Part model, mm, in its own coordinate system. A direction names the side the tool comes from. Round coordinates to 2 decimals unless told otherwise and drop trailing zeros. Order: outer loops, then holes, each group sorted by start corner. A loop starts at its lowest first (then second) coordinate and runs counter-clockwise, first axis right, second up. Notation, with made-up numbers: (-34.5, 61.5) -> (1.5, 61.5) arc R11 ccw to (1.5, 79.5) -> close; hole circle Ø3 at (44, 38.25). An arc over 180 degrees is marked (long way). Use CSV: the item, a comma, the result in double quotes.
```python
from build123d import *

# Parameters (mm, degrees)
EXTRUDE1_DEPTH     = 304.8
SKETCH2_R          = 1.5875
EXTRUDE2_DEPTH     = 1.5875
SKETCH3_R          = 1.5875
CUT_EXTRUDE3_DEPTH = 306.9883086
SKETCH6_R          = 1.5875
CUT_EXTRUDE5_DEPTH = 306.9883086
SKETCH7_W          = 17.4625
SKETCH7_H          = 11.77006403
CUT_EXTRUDE6_DEPTH = 306.893578563


with BuildPart() as part:
    # Sketch1 → Extrude1 (new body)
    with BuildSketch(Plane.XY):
        Polygon((0, 0), (0, 19.05), (-1.5875, 19.05), (-1.5875, 1.5875), (-19.05, 1.5875), (-19.05, 0), align=None)
    extrude(amount=EXTRUDE1_DEPTH)

    # Sketch2 → Extrude2 (cut)
    with BuildSketch(Plane(origin=(0, 0, 0), x_dir=(0, 0, -1), z_dir=(1, 0, 0))):
        with Locations((-298.45, 9.525)):
            Circle(SKETCH2_R)
        with Locations((-234.95, 9.525)):
            Circle(SKETCH2_R)
    extrude(amount=-EXTRUDE2_DEPTH, mode=Mode.SUBTRACT)

    # Sketch3 → Cut-Extrude3 (cut, through all)
    with BuildSketch(Plane(origin=(0, 0, 0), x_dir=(0, 0, -1), z_dir=(1, 0, 0))):
        with Locations((-26.555576272, 9.525)):
            Circle(SKETCH3_R)
        with Locations((-16.452788136, 9.525)):
            Circle(SKETCH3_R)
    extrude(amount=-CUT_EXTRUDE3_DEPTH, mode=Mode.SUBTRACT)

    # Sketch6 → Cut-Extrude5 (cut, through all)
    with BuildSketch(Plane(origin=(0, 0, 0), x_dir=(0, 0, -1), z_dir=(1, 0, 0))):
        with Locations((-8.59506403, 15.875)):
            Circle(SKETCH6_R)
        with Locations((-8.59506403, 3.175)):
            Circle(SKETCH6_R)
        with Locations((-6.35, 9.525)):
            Circle(SKETCH6_R)
    extrude(amount=-CUT_EXTRUDE5_DEPTH, mode=Mode.SUBTRACT)

    # Sketch7 → Cut-Extrude6 (cut, through all)
    with BuildSketch(Plane(origin=(0, 1.5875, 0), x_dir=(1, 0, 0), z_dir=(0, 1, 0))):
        with Locations((-10.31875, -5.885032015)):
            Rectangle(SKETCH7_W, SKETCH7_H)
    extrude(amount=-CUT_EXTRUDE6_DEPTH, mode=Mode.SUBTRACT)


solid = part.part
```
(1) Cut at A-A, the plane z = 157.5. Give the cut face in (x, y), then the cut area to 3 significant figures.
Reply:
outline,"(-19.05, 0) -> (0, 0) -> (0, 19.05) -> (-1.59, 19.05) -> (-1.59, 1.59) -> (-19.05, 1.59) -> close"
area,"58.0 mm2"
(2) Which spindle directions (+Z, -Z, +X, -X, +Y, -Y) get a long thin tool onto all of the face, cutting with end or side? Do faces 1 (the face through (-5, 1, 304.8)), 2 (the face through (-10, 1.588, 156)). Say none if no direction does.
Reply:
face 1,"+Z, +X, -X, +Y, -Y"
face 2,"+Z, -Z, -X, +Y"
(3) Probe probe 1 along Y at (x, z) = (-5, 194.5); probe 2 along X at (y, z) = (15, 234); probe 3 along Z at (x, y) = (-9.75, 1). List the from-to ranges inside material, lowest first. Write a range as [from, to].
Reply:
probe 1,"[0, 1.59]"
probe 2,"[-1.59, 0]"
probe 3,"[11.77, 304.8]"
(4) Drop flat-ended pins along their axis: P1, Ø8, axis at x = -12, y = 4, coming from the -Z side; P2, Ø5, axis at y = 9.525, z = 6.35, coming from the -X side; P3, Ø1.9, axis at y = 9.525, z = 298.45, coming from the -X side. Give the stop position or say it passes through.
Reply:
P1,"z = 11.77"
P2,"x = -1.59"
P3,"through"
(5) Cut at B-B, the plane x = -13. Give the cut face in (y, z), then the cut area to 3 significant figures.
Reply:
outline,"(0, 11.77) -> (1.59, 11.77) -> (1.59, 304.8) -> (0, 304.8) -> close"
area,"465 mm2"
